```python
from build123d import *

# Parameters (mm, degrees)
SKETCH1_R           = 11
BOSS_EXTRUDE1_DEPTH = 2
SKETCH2_R           = 7
BOSS_EXTRUDE2_DEPTH = 2.2
SKETCH3_R           = 5.5
BOSS_EXTRUDE3_DEPTH = 1
BOSS_EXTRUDE4_DEPTH = 0.4
BOSS_EXTRUDE5_DEPTH = 3


with BuildPart() as part:
    # Sketch1 → Boss-Extrude1 (new body)
    with BuildSketch(Plane.XY):
        Circle(SKETCH1_R)
    extrude(amount=BOSS_EXTRUDE1_DEPTH)

    # Sketch2 → Boss-Extrude2 (add)
    with BuildSketch(Plane(origin=(0, 0, 0), x_dir=(-1, 0, 0), z_dir=(0, 0, -1))):
        with Locations(Location((0, 0, 0), (0, 0, 180))):
            Circle(SKETCH2_R)
    extrude(amount=BOSS_EXTRUDE2_DEPTH)

    # Sketch3 → Boss-Extrude3 (add)
    with BuildSketch(Plane(origin=(0, 0, -2.2), x_dir=(-1, 0, 0), z_dir=(0, 0, -1))):
        Circle(SKETCH3_R)
    extrude(amount=BOSS_EXTRUDE3_DEPTH)

    # Sketch4 → Boss-Extrude4 (add)
    with BuildSketch(Plane(origin=(0, 0, -3.2), x_dir=(-1, 0, 0), z_dir=(0, 0, -1))):
        Polygon((-4, 3.774917218), (4, 3.774917218), (8.6, -5), (8.6, -18), (7.6, -18), (6.9, -11), (5.1, -11), (5.1, -2.059126028), (3.85, -2.059126028), (3.5, -18), (2.5, -18), (2.15, -2.059126028), (0.85, -2.059126028), (0.5, -18), (-0.5, -18), (-0.85, -2.059126028), (-2.15, -2.059126028), (-2.5, -18), (-3.5, -18), (-3.85, -2.059126028), (-5.1, -2.059126028), (-5.1, -11), (-6.9, -11), (-7.6, -18), (-8.6, -18), (-8.6, -5), align=None)
    extrude(amount=BOSS_EXTRUDE4_DEPTH)

    # Sketch5 → Boss-Extrude5 (add)
    with BuildSketch(Plane(origin=(0, 0, -3.6), x_dir=(-1, 0, 0), z_dir=(0, 0, -1))):
        Polygon((-8.6, -5), (-4, 3.774917218), (4, 3.774917218), (8.6, -5), align=None)
    extrude(amount=BOSS_EXTRUDE5_DEPTH)


solid = part.part
```
Source: CAD feature listing. Evaluate the final solid. Frame: model axes, mm. A direction names the side the tool comes from. Give positions to 0.01 mm unless a question says otherwise; leave off trailing zeros. Order: outer loops, then holes, each group sorted by start corner. A loop starts at its lowest first (then second) coordinate and runs counter-clockwise, first axis right, second up.
(1) Section query B-B (x = 0). Return the cut outline in (y, z), plus the area to 3 significant figures.
(2) Access query for faces 1 (the face through (0, 4, -3.2)), 2 (the face through (0, -11, -3.6)), 3 (the face through (-4, -3, -3.2)), 4 (the face through (6.466, 2.681, -1.085)), 5 (the face through (0, -12, -3.2)). Directions: +Z, -Z, +X, -X, +Y, -Y. A direction counts if a zero-diameter tool reaches every point of the face in a straight line with its end or side. Return the directions, or none.
(3) Section query D-D (y = 0). Return the cut outline in (x, z), plus the area to 3 significant figures.
(4) Section query C-C (y = -8.75). Return the cut outline in (x, z), plus the area to 3 significant figures.
(5) Material intervals for line 1 along X through (y, z) = (-11.5, -3.5); line 2 along Z through (x, y) = (-5, -9); line 3 along Z through (x, y) = (5.5, 2), sorted ascending.
(6) Section query A-A (y = -14.25). Return the cut outline in (x, z) (3 decimals), plus the area to 3 significant figures.
(7) Contact query for flat-ended pins moving along their axis: P1, Ø2, axis at y = -9, z = -3, coming from the +X side; P2, Ø3.5, axis at x = -2.5, z = -5.5, coming from the -Y side; P3, Ø0.5, axis at x = 1.5, y = 4.5, coming from the -Z side. Output: stop coordinate, or through.
Outcome:
1. outline: (-18, -3.6) - (-5, -3.6) - (-5, -6.6) - (3.77, -6.6) - (3.77, -3.2) - (5.5, -3.2) - (5.5, -2.2) - (7, -2.2) - (7, 0) - (11, 0) - (11, 2) - (-11, 2) - (-11, 0) - (-7, 0) - (-7, -2.2) - (-5.5, -2.2) - (-5.5, -3.2) - (-18, -3.2) - close
1. area: 121 mm2
2. face 1: -Z, +X, -X, +Y
2. face 2: -Z, +X, -X, -Y
2. face 3: -Y
2. face 4: none
2. face 5: +X, -X, -Y
3. outline: (-11, 0) - (-7, 0) - (-7, -2.2) - (-5.5, -2.2) - (-5.5, -3.2) - (-5.98, -3.2) - (-5.98, -6.6) - (5.98, -6.6) - (5.98, -3.2) - (5.5, -3.2) - (5.5, -2.2) - (7, -2.2) - (7, 0) - (11, 0) - (11, 2) - (-11, 2) - close
3. area: 126 mm2
4. outline: (-8.6, -3.6) - (-5.1, -3.6) - (-5.1, -3.2) - (-8.6, -3.2) - close; (-6.67, 0) - (6.67, 0) - (6.67, 2) - (-6.67, 2) - close; (-3.7, -3.6) - (-2.3, -3.6) - (-2.3, -3.2) - (-3.7, -3.2) - close; (-0.7, -3.6) - (0.7, -3.6) - (0.7, -3.2) - (-0.7, -3.2) - close; (2.3, -3.6) - (3.7, -3.6) - (3.7, -3.2) - (2.3, -3.2) - close; (5.1, -3.6) - (8.6, -3.6) - (8.6, -3.2) - (5.1, -3.2) - close
4. area: 31.2 mm2
5. line 1: x = -8.6 to -6.95, -3.64 to -2.36, -0.64 to 0.64, 2.36 to 3.64, 6.95 to 8.6
5. line 2: z = 0 to 2
5. line 3: z = -2.2 to 2
6. outline: (-8.6, -3.6) - (-7.225, -3.6) - (-7.225, -3.2) - (-8.6, -3.2) - close; (-3.582, -3.6) - (-2.418, -3.6) - (-2.418, -3.2) - (-3.582, -3.2) - close; (-0.582, -3.6) - (0.582, -3.6) - (0.582, -3.2) - (-0.582, -3.2) - close; (2.418, -3.6) - (3.582, -3.6) - (3.582, -3.2) - (2.418, -3.2) - close; (7.225, -3.6) - (8.6, -3.6) - (8.6, -3.2) - (7.225, -3.2) - close
6. area: 2.50 mm2
7. P1: stops at x = 8.6
7. P2: stops at y = -5
7. P3: stops at z = -3.2
